Check sheet for the drawn part. Datum: minimum x, y, z corner. Units: mm. A direction names the side the tool comes from. Coordinates: 2 decimals unless noted, no trailing zeros. Order: outer loops, then holes, each group sorted by start corner. A loop starts at its lowest first (then second) coordinate and runs counter-clockwise, first axis right, second up. Notation, with made-up numbers: (-6, 68) - (15, 68) arc R14 ccw to (15, 88) - close; hole circle Ø5 at (37.5, -17). An arc over 180 degrees is marked (long way). Return JSON: item names as keys, results as strings. Group by question number.
Item 1: Scan lines: probe 1 along X at (y, z) = (4.75, 4); probe 2 along X at (y, z) = (13.25, 1.5); probe 3 along Z at (x, y) = (5.25, 12). Record each from-to range of solid material in increasing order.
Item 2: Section check B-B on z = 5.5. Enter the section's corners in (x, y), then the cut area to 3 significant figures.
Item 3: Draft check along X on the marked faces 1, 2 and 3. Enter one of: pulls with the +X half, pulls with the -X half, needs draft (parallel to the pull), parting line crosses it, or undercut.
Item 4: Tool access check on the marked faces 4 and 5. Record the directions out of +Z, -Z, +X, -X, +Y, -Y that give a thin tool (end or side, any length) a straight path to the whole face; none if there is none.
Item 5: Section check D-D on x = 7.25. Enter the section's corners in (y, z) (3 decimals).
Item 6: Section check A-A on x = 4.75. Enter the section's corners in (y, z).
Item 7: Section check C-C on y = 9. Enter the section's corners in (x, z) (3 decimals), then the cut area to 3 significant figures.
Item 8: Gauge pin test, flat ends, axial feed: pin 1 (1.5 mm diameter, centred on x = 5.5, y = 8.5, fed in from -Z); pin 2 (1.5 mm diameter, centred on x = 5.5, z = 5, fed in from +Y); pin 3 (2 mm diameter, centred on x = 3, z = 6.5, fed in from -Y); pin 4 (0.6 mm diameter, centred on x = 7, y = 1, fed in from +Z). Record the tip position at first contact, or that the pin passes through.
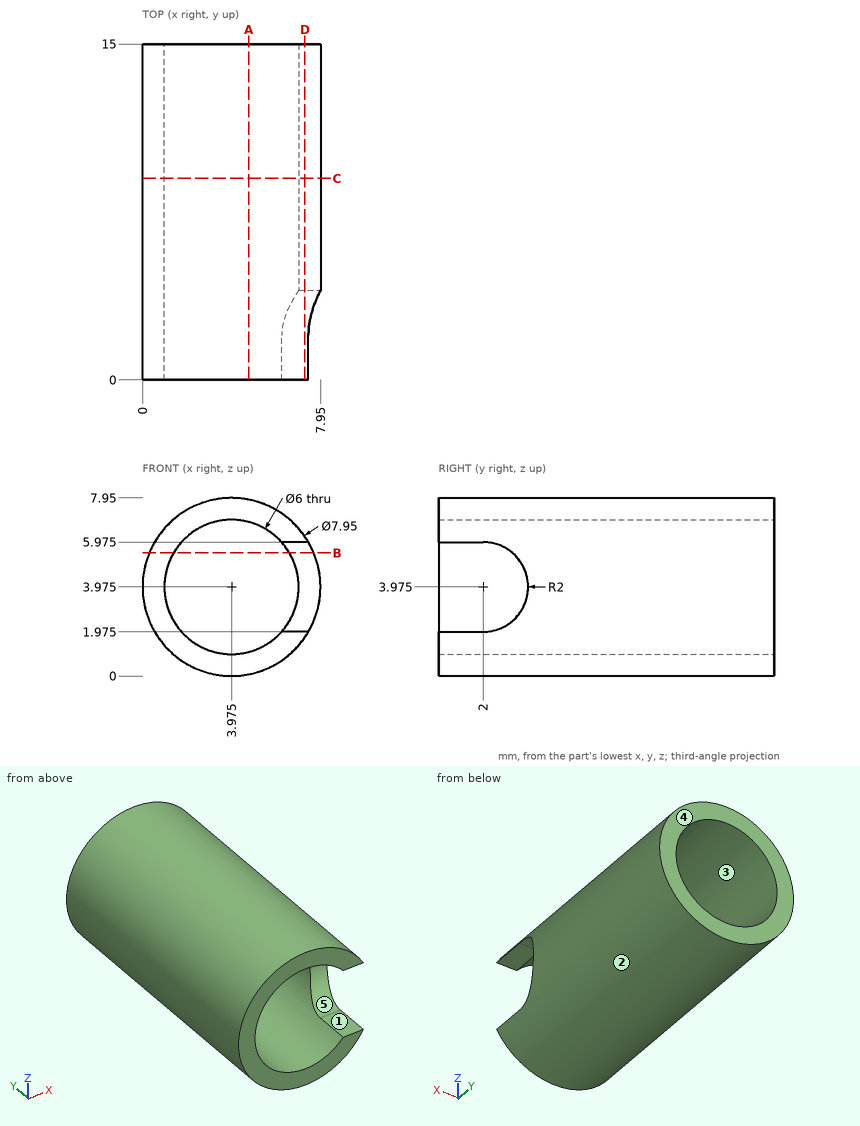
Computed:
{
 "1": {"probe 1": "x = 0 to 0.98, 6.97 to 7.95", "probe 2": "x = 0.86 to 2.28, 5.67 to 7.09", "probe 3": "z = 0.21 to 1.26, 6.69 to 7.74"},
 "2": {"outline": "(0.3, 0) - (1.39, 0) - (1.39, 15) - (0.3, 15) - close; (6.56, 3.29) - (7.65, 3.29) - (7.65, 15) - (6.56, 15) - close", "area": "29.0 mm²"},
 "3": {"face 1": "needs draft", "face 2": "parting line crosses it", "face 3": "undercut"},
 "4": {"face 4": "+Z, -Z, +X, -X, +Y", "face 5": "+X, -Y"},
 "5": {"outline": "(0, 1.722) - (15, 1.722) - (15, 6.228) - (0, 6.228) - (0, 5.975) - (2, 5.975) arc R2 cw to (2, 1.975) - (0, 1.975) - close"},
 "6": {"outline": "(0, 0.08) - (15, 0.08) - (15, 1.08) - (0, 1.08) - close; (0, 6.87) - (15, 6.87) - (15, 7.87) - (0, 7.87) - close"},
 "7": {"outline": "circle Ø7.95 at (3.975, 3.975); hole circle Ø6 at (3.975, 3.975)", "area": "21.4 mm²"},
 "8": {"pin 1": "stops at z = 0.08", "pin 2": "passes through", "pin 3": "stops at y = 0", "pin 4": "stops at z = 6.87"}
}
